```python
from build123d import *
from OCP.BRepFilletAPI import BRepFilletAPI_MakeChamfer
from build123d.topology import SkipClean

# Parameters (mm, degrees)
CROQUIS1_W              = 98
CROQUIS1_H              = 60
SALIENTE_EXTRUIR1_DEPTH = 1
CROQUIS2_W              = 12.2
CROQUIS2_H              = 18
SALIENTE_EXTRUIR2_DEPTH = 10
SALIENTE_EXTRUIR3_START = -88
CROQUIS2_3_W            = 12.2
CROQUIS2_3_H            = 18
SALIENTE_EXTRUIR3_DEPTH = 10
CORTAR_EXTRUIR1_DEPTH   = 115
CORTAR_EXTRUIR2_DEPTH   = 115
REDONDEO1_R             = 10
REDONDEO2_START         = -43
REDONDEO2_DEPTH         = 100
CROQUIS4_R              = 1.624451876
CROQUIS4_W              = 8
CROQUIS4_H              = 6
CORTAR_EXTRUIR3_DEPTH   = 41
SALIENTE_EXTRUIR4_DEPTH = 5
CHAFL_N1_SIZE           = 5
CHAFL_N1_SIZE_2         = 2.020131129
CORTAR_EXTRUIR4_DEPTH   = 101
SALIENTE_EXTRUIR5_DEPTH = 26
SALIENTE_EXTRUIR6_START = -72
SALIENTE_EXTRUIR6_DEPTH = 26
CORTAR_EXTRUIR5_DEPTH   = 72
SALIENTE_EXTRUIR7_START = -88
CROQUIS7_5_W            = 2
CROQUIS7_5_H            = 4.363894299
SALIENTE_EXTRUIR7_DEPTH = 78


with BuildPart() as part:
    # Croquis1 → Saliente-Extruir1 (new body)
    with BuildSketch(Plane(origin=(0, 0, 0), x_dir=(1, 0, 0), z_dir=(0, 1, 0))):
        with Locations((7.309859155, 2.323943662)):
            Rectangle(CROQUIS1_W, CROQUIS1_H)
    extrude(amount=SALIENTE_EXTRUIR1_DEPTH)

    # Croquis2 → Saliente-Extruir2 (add)
    with BuildSketch(Plane.ZY.offset(41.690140845)):
        with BuildLine():
            Line((-22.673615367, 7.404257104), (-31.02059504, 1))
            Line((-31.02059504, 1), (27.676056338, 1))
            Line((27.676056338, 1), (27.676056338, 1.85662729))
            ThreePointArc((27.676056338, 1.85662729), (25.837285222, 8.581073785), (27.676056338, 15.305520281))
            Line((27.676056338, 15.305520281), (27.676056338, 22))
            Line((27.676056338, 22), (-14.080479284, 22))
            Line((-14.080479284, 22), (-22.673615367, 7.404257104))
        make_face()
        with Locations((6.911108061, 10.408932756)):
            Rectangle(CROQUIS2_W, CROQUIS2_H, mode=Mode.SUBTRACT)
    extrude(amount=-SALIENTE_EXTRUIR2_DEPTH)

    # Croquis2<3> → Saliente-Extruir3 (add)
    with BuildSketch(Plane.ZY.offset(41.690140845).offset(SALIENTE_EXTRUIR3_START)):
        with BuildLine():
            Line((-22.673615367, 7.404257104), (-31.02059504, 1))
            Line((-31.02059504, 1), (27.676056338, 1))
            Line((27.676056338, 1), (27.676056338, 1.85662729))
            ThreePointArc((27.676056338, 1.85662729), (25.837285222, 8.581073785), (27.676056338, 15.305520281))
            Line((27.676056338, 15.305520281), (27.676056338, 22))
            Line((27.676056338, 22), (-14.080479284, 22))
            Line((-14.080479284, 22), (-22.673615367, 7.404257104))
        make_face()
        with Locations((6.911108061, 10.408932756)):
            Rectangle(CROQUIS2_3_W, CROQUIS2_3_H, mode=Mode.SUBTRACT)
    extrude(amount=-SALIENTE_EXTRUIR3_DEPTH)

    # Croquis2<4> → Cortar-Extruir1 (cut)
    with BuildSketch(Plane.ZY.offset(41.690140845)):
        Polygon((-32.323943662, 1), (-32.323943662, 0), (-31.02059504, 1), align=None)
    extrude(amount=-CORTAR_EXTRUIR1_DEPTH, mode=Mode.SUBTRACT)

    # Croquis3 → Cortar-Extruir2 (cut)
    with BuildSketch(Plane(origin=(0, 1, 0), x_dir=(1, 0, 0), z_dir=(0, 1, 0))):
        Polygon((-40.291413083, 31.02059504), (-31.690140845, 9.370184618), (-31.690140845, 31.02059504), align=None)
        Polygon((54.911131393, 31.02059504), (46.309859155, 31.02059504), (46.309859155, 9.370184618), align=None)
    extrude(amount=CORTAR_EXTRUIR2_DEPTH, mode=Mode.SUBTRACT)

    # Redondeo1
    # the kernel refuses this fillet: 10 mm, written as the material it takes off along each edge
    # the kernel refuses this fillet: 10 mm, written as the material it takes off along each edge
    with BuildSketch(Plane(origin=(-46.33170907, 1.85662729, 27.676056338), x_dir=(0, 0.8924889538837264, -0.4510692487806408), z_dir=(1, 0, 0))) as redondeo1_2_piece_1:
        with BuildLine():
            CenterArc((2.398228131, -9.978308132), REDONDEO1_R, 93.774545272, 20.149469447)
            Line((-1.657019348, -0.837467477), (0, 0))
            ThreePointArc((0, 0), (0.869961056, -0.028666121), (1.739922113, 0))
        make_face()
    extrude(amount=19.283136451, mode=Mode.SUBTRACT)
    # the kernel refuses this fillet: 10 mm, written as the material it takes off along each edge
    # the kernel refuses this fillet: 10 mm, written as the material it takes off along each edge
    with BuildSketch(Plane(origin=(41.66829093, 1.85662729, 27.676056338), x_dir=(0, -1, 0), z_dir=(1, 0, 0))) as redondeo1_4_piece_1:
        with BuildLine():
            CenterArc((2.360515838, 9.987296748), REDONDEO1_R, 246.962238713, 20.149469447)
            ThreePointArc((-1.552861266, 0.78482536), (-0.763500227, 0.417996876), (0, 0))
            Line((0, 0), (1.85662729, 0))
        make_face()
    extrude(amount=19.283136451, mode=Mode.SUBTRACT)
    # the kernel refuses this fillet: 10 mm, written as the material it takes off along each edge
    with BuildSketch(Plane(origin=(52.565538288, 1, 27.676056338), x_dir=(0, -1, 0), z_dir=(-1, 0, 0))) as redondeo1_5_piece_1_section:
        with BuildLine():
            CenterArc((10, -4.358898944), REDONDEO1_R, 154.158067237, 25.841932763)
            Line((0, -4.358898944), (0, 0))
            Line((0, 0), (1, 0))
        make_face()
    redondeo1_5_piece_1 = extrude(amount=90.511358267, mode=Mode.PRIVATE)
    redondeo1_5_piece_1 = redondeo1_5_piece_1 - Plane(origin=(52.565538288, -0.503888548, 17.68875959), x_dir=(0, 0.050388854784132256, 0.998729674793707), z_dir=(-1, 0, 0)) * Cylinder(10, 199, mode=Mode.PRIVATE)
    add(redondeo1_5_piece_1, mode=Mode.SUBTRACT)

    # Redondeo2: read off the stored shape, not the designer's step
    # Redondeo2 outline → Redondeo2 (cut)
    with SkipClean():  # the faces are left unmerged after this step: merging them gives an invalid solid
        with BuildSketch(Plane.YZ.offset(REDONDEO2_START)):
            with BuildLine():
                ThreePointArc((13.735621222, 26.883999693), (15.646059665, 27.476041888), (17.636105701, 27.676056338))
                Line((17.636105701, 27.676056338), (15.305520281, 27.676056338))
                ThreePointArc((15.305520281, 27.676056338), (14.533759116, 27.253887965), (13.735621222, 26.883999693))
            make_face()
        extrude(amount=REDONDEO2_DEPTH, mode=Mode.SUBTRACT)
    add(part.part.scale(1), mode=Mode.REPLACE)  # the faces are merged on a copy

    # Croquis4 → Cortar-Extruir3 (cut)
    with BuildSketch(Plane.XZ):
        with Locations(Location((-37.960140845, 17.674595399, 0), (0, 0, 270))):
            Circle(CROQUIS4_R)
        with Locations(Location((52.579859155, 17.674595399, 0), (0, 0, 270))):
            Circle(CROQUIS4_R)
        with Locations((-25.233647173, -20.164268386)):
            Rectangle(CROQUIS4_W, CROQUIS4_H)
        with Locations((39.853365482, -20.164268386)):
            Rectangle(CROQUIS4_W, CROQUIS4_H)
    extrude(amount=-CORTAR_EXTRUIR3_DEPTH, mode=Mode.SUBTRACT)

    # Croquis5 → Saliente-Extruir4 (add)
    with BuildSketch(Plane(origin=(0, 1, 0), x_dir=(1, 0, 0), z_dir=(0, 1, 0))):
        Polygon((-1.913897366, 6.29786762), (-1.913897366, 18.591303013), (-8.5088233, 18.784914739), (-5.73410883, 6.29786762), align=None)
        Polygon((-9.811245677, 6.29786762), (-12.612731972, 18.905395977), (-16.070794085, 19.006916659), (-11.021744735, 6.29786762), align=None)
        Polygon((16.533615676, 18.591303013), (16.533615676, 6.29786762), (20.35382714, 6.29786762), (23.12854161, 18.784914739), align=None)
        Polygon((27.232450282, 18.905395977), (24.430963987, 6.29786762), (25.641463045, 6.29786762), (30.690512395, 19.006916659), align=None)
    extrude(amount=SALIENTE_EXTRUIR4_DEPTH)

    # Chaflán1
    chafl_n1_edges_1 = [part.edges().sort_by_distance(p)[0] for p in [
        (25.831707134, 6, -12.601631799),
    ]]
    chafl_n1_side_1 = [part.faces().sort_by_distance(p)[0] for p in [
        (25.831707134, 5.959597377, -12.601631799),
    ]]
    chafl_n1_edges_2 = [part.edges().sort_by_distance(p)[0] for p in [
        (21.741184375, 6, -12.541391179),
    ]]
    chafl_n1_side_2 = [part.faces().sort_by_distance(p)[0] for p in [
        (21.741184375, 5.959597377, -12.541391179),
    ]]
    chafl_n1_edges_3 = [part.edges().sort_by_distance(p)[0] for p in [
        (-11.211988825, 6, -12.601631799),
    ]]
    chafl_n1_side_3 = [part.faces().sort_by_distance(p)[0] for p in [
        (-11.211988825, 5.959597377, -12.601631799),
    ]]
    chafl_n1_edges_4 = [part.edges().sort_by_distance(p)[0] for p in [
        (-7.121466065, 6, -12.541391179),
    ]]
    chafl_n1_side_4 = [part.faces().sort_by_distance(p)[0] for p in [
        (-7.121466065, 5.959597377, -12.541391179),
    ]]
    chafl_n1 = BRepFilletAPI_MakeChamfer(part.part.solid().wrapped)
    for e in chafl_n1_edges_1:
        chafl_n1.Add(CHAFL_N1_SIZE - 0.0001, CHAFL_N1_SIZE_2 - 0.0001, e.wrapped, chafl_n1_side_1[0].wrapped)
    for e in chafl_n1_edges_2:
        chafl_n1.Add(CHAFL_N1_SIZE - 0.0001, CHAFL_N1_SIZE_2 - 0.0001, e.wrapped, chafl_n1_side_2[0].wrapped)
    for e in chafl_n1_edges_3:
        chafl_n1.Add(CHAFL_N1_SIZE - 0.0001, CHAFL_N1_SIZE_2 - 0.0001, e.wrapped, chafl_n1_side_3[0].wrapped)
    for e in chafl_n1_edges_4:
        chafl_n1.Add(CHAFL_N1_SIZE - 0.0001, CHAFL_N1_SIZE_2 - 0.0001, e.wrapped, chafl_n1_side_4[0].wrapped)
    add(Compound.cast(chafl_n1.Shape()), mode=Mode.REPLACE)  # a hair under: the kernel refuses the full size

    # Croquis6 → Cortar-Extruir4 (cut)
    with BuildSketch(Plane.ZY.offset(41.690140845)):
        Polygon((-22.673615367, 7.404257104), (-31.323943662, 0), (-32.323943662, 0), align=None)
    extrude(amount=-CORTAR_EXTRUIR4_DEPTH, mode=Mode.SUBTRACT)

    # Croquis7 → Saliente-Extruir5 (add)
    with BuildSketch(Plane.ZY.offset(41.690140845)):
        with BuildLine():
            Line((27.676056338, 17.636105701), (25.676056338, 17.636105701))
            ThreePointArc((25.676056338, 17.636105701), (25.516044778, 16.044068872), (25.042411022, 14.515718118))
            ThreePointArc((25.042411022, 14.515718118), (23.837288952, 8.570418777), (25.0507367, 2.626813135))
            ThreePointArc((25.0507367, 2.626813135), (25.473403095, 1.339837436), (25.67287484, 0))
            Line((25.67287484, 0), (27.676056338, 0))
            ThreePointArc((27.676056338, 0), (27.433909837, 1.739333838), (26.891230978, 3.409488556))
            ThreePointArc((26.891230978, 3.409488556), (25.837288462, 8.571819356), (26.883999693, 13.735621222))
            ThreePointArc((26.883999693, 13.735621222), (27.476041888, 15.646059665), (27.676056338, 17.636105701))
        make_face()
    extrude(amount=-SALIENTE_EXTRUIR5_DEPTH)

    # Croquis7<4> → Saliente-Extruir6 (add)
    with BuildSketch(Plane.ZY.offset(41.690140845).offset(SALIENTE_EXTRUIR6_START)):
        with BuildLine():
            Line((27.676056338, 17.636105701), (25.676056338, 17.636105701))
            ThreePointArc((25.676056338, 17.636105701), (25.516044778, 16.044068872), (25.042411022, 14.515718118))
            ThreePointArc((25.042411022, 14.515718118), (23.837288952, 8.570418777), (25.0507367, 2.626813135))
            ThreePointArc((25.0507367, 2.626813135), (25.473403095, 1.339837436), (25.67287484, 0))
            Line((25.67287484, 0), (27.676056338, 0))
            ThreePointArc((27.676056338, 0), (27.433909837, 1.739333838), (26.891230978, 3.409488556))
            ThreePointArc((26.891230978, 3.409488556), (25.837288462, 8.571819356), (26.883999693, 13.735621222))
            ThreePointArc((26.883999693, 13.735621222), (27.476041888, 15.646059665), (27.676056338, 17.636105701))
        make_face()
    extrude(amount=-SALIENTE_EXTRUIR6_DEPTH)

    # Croquis8 → Cortar-Extruir5 (cut)
    with BuildSketch(Plane.XY.offset(27.676056338)):
        Polygon((-43.181006637, 23.333071417), (-41.690140845, 1), (-35.872500086, 17.636105701), (-41.690140845, 17.636105701), (-41.690140845, 22), (-34.346447667, 22), align=None)
        Polygon((-41.690140845, 17.636105701), (-35.872500086, 17.636105701), (-34.346447667, 22), (-41.690140845, 22), align=None)
        Polygon((57.800724947, 23.333071417), (56.309859155, 1), (48.966165977, 22), align=None)
    extrude(amount=-CORTAR_EXTRUIR5_DEPTH, mode=Mode.SUBTRACT)

    # Croquis7<5> → Saliente-Extruir7 (add)
    with BuildSketch(Plane.ZY.offset(41.690140845).offset(SALIENTE_EXTRUIR7_START)):
        with Locations((26.676056338, 19.818052851)):
            Rectangle(CROQUIS7_5_W, CROQUIS7_5_H)
    extrude(amount=SALIENTE_EXTRUIR7_DEPTH)


solid = part.part
```
Here's how the part is built. I have some questions about the finished solid (model axes, mm). A direction names the side the tool comes from. Coordinates: 2 decimals unless noted, no trailing zeros. Write each loop counter-clockwise with the first axis right and the second up, starting at its lowest first coordinate (ties: lowest second). Pieces come first, ordered by that corner, then holes. Notation, with made-up numbers: M 76.5,57 L 90.5,57 A24 ccw 90.5,90 Z; hole C -14.75,-14.5 d9. An arc over 180 degrees is marked long. Answer as CSV lines item,"result". Start each with the question number.
Q1. Suppose I cut it at A-A, the plane x = 41. List the corners of the cut face in (y, z) for me.
Q2. Suppose I cut it at D-D, the plane z = 17. List the corners of the cut face in (x, y) for me, then the cut area to 3 significant figures.
Q3. I need wall thicknesses on probe 1 along Y at (x, z) = (23.5, -19); probe 2 along Z at (x, y) = (-26.5, 8); probe 3 along X at (y, z) = (3, 23). Which ranges of each line are inside material? Lowest first, please. Write a range as [from, to].
Q4. Suppose I cut it at B-B, the plane y = 8.75. List the corners of the cut face in (x, z) for me.
Q5. Suppose I cut it at C-C, the plane z = -2. List the corners of the cut face in (x, y) for me.
Q6. For faces 4 (the flat face through (51, 1.409, 7)), 5 (the flat face through (8, 17.636, 27)), 6 (the flat face through (26.91, 3.54, -12.72)), which set-ups out of +Z, -Z, +X, -X, +Y, -Y let a thin tool reach every point of the face, with its end or its side?
Q7. If we mould it in two halves opening along Z, with no side actions, what happens to faces 1 (the cylindrical face through (6.62, 0.56, 27.63)), 2 (the flat face through (8, 22, 27)), 3 (the flat face through (48, 19.409, 7))? For each: pulls with the +Z half, pulls with the -Z half, needs draft (parallel to the pull), parting line crosses it, or undercut.
Q8. Will these pins go through, and if not, where does the flat tip stop? pin 1 Ø0.8 at (x, y) = (38, 0.5) entering from -Z; pin 2 Ø1 at (y, z) = (17, 13.5) entering from +X; pin 3 Ø3 at (x, y) = (-4, 3.5) entering from +Z; pin 4 Ø10.5 at (y, z) = (13.5, 7) entering from +X.
Entries:
1,outline,"M 0,-31.32 L 1,-30.16 L 1,-23.16 L 0,-23.16 Z; M 0,-17.16 L 1,-17.16 L 1,25.55 A8 cw 2.63,25.05 A15.22 ccw 14.52,25.04 A8 cw 17.64,25.68 L 22,25.68 L 22,27.68 L 17.64,27.68 A10 ccw 13.74,26.88 A13.22 cw 3.41,26.89 A10 ccw 0,27.68 Z"
2,outline,"M -41.69,0 L -39.44,0 L -39.44,7.44 L -41.69,1 Z; M -36.48,0 L 51.1,0 L 51.1,15.89 L 48.97,22 L 46.31,22 L 46.31,1 L -31.69,1 L -31.69,22 L -34.35,22 L -36.48,15.89 Z; M 54.06,0 L 56.31,0 L 56.31,1 L 54.06,7.44 Z"
2,area,"295 mm²"
3,probe 1,"y = [0, 1]"
3,probe 2,"z = [23.85, 25.85]"
3,probe 3,"x = [-40.99, -31.69], [46.31, 55.61]"
4,outline,"M -38.98,-21.88 L -36.66,-21.88 L -31.69,-9.37 L -31.69,0.81 L -38.98,0.81 Z; M -38.98,13.01 L -31.69,13.01 L -31.69,23.84 L -15.69,23.84 L -15.69,25.84 L -38.98,25.84 L -38.98,18.94 A1.62 cw long -38.98,16.41 Z; M 30.31,23.84 L 46.31,23.84 L 46.31,13.01 L 53.6,13.01 L 53.6,16.41 A1.62 cw long 53.6,18.94 L 53.6,25.84 L 30.31,25.84 Z; M 46.31,-9.37 L 51.28,-21.88 L 53.6,-21.88 L 53.6,0.81 L 46.31,0.81 Z"
5,outline,"M -41.69,0 L 56.31,0 L 56.31,1 L 48.97,22 L 46.31,22 L 46.31,1 L -31.69,1 L -31.69,22 L -34.35,22 L -41.69,1 Z"
6,face 4,"+X, -X"
6,face 5,"+Z, -Z"
6,face 6,"-Z, +Y"
7,face 1,"pulls with the +Z half"
7,face 2,"needs draft"
7,face 3,"undercut"
8,pin 1,"stops at z = -31.21"
8,pin 2,"stops at x = 50.89"
8,pin 3,"stops at z = -6.3"
8,pin 4,"passes through"
